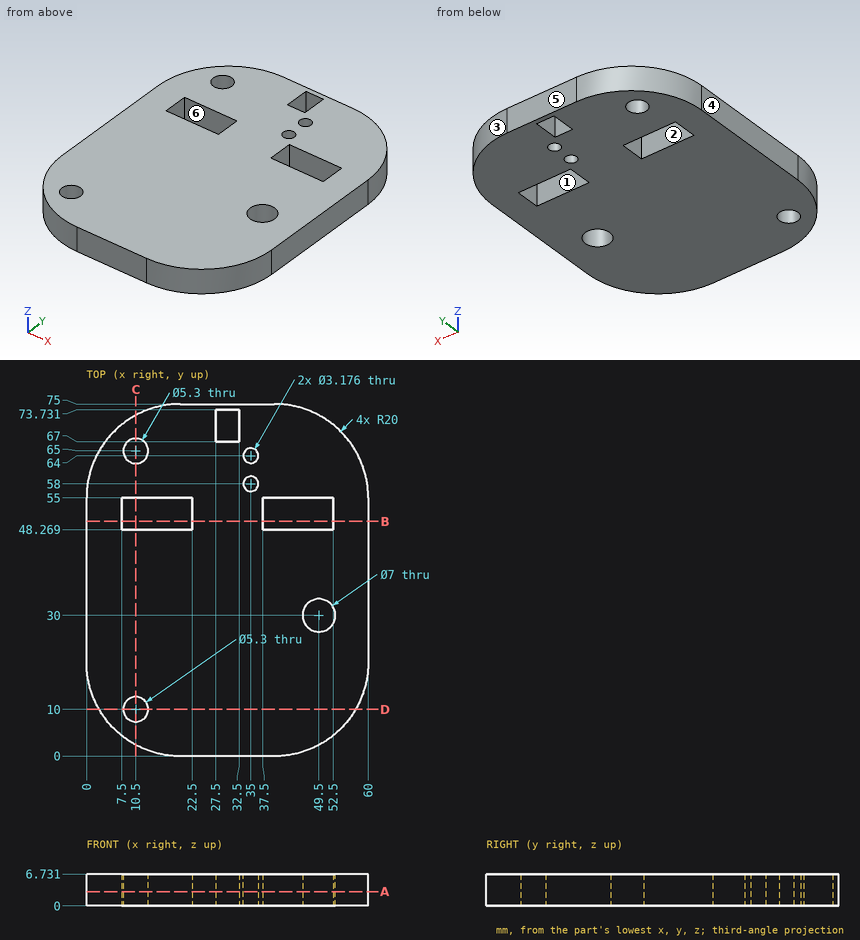
Answer from the drawing. Dimensions are ordinates in mm from the lowest x, y and z of the part. A direction names the side the tool comes from. Give positions to 0.01 mm unless a question says otherwise; leave off trailing zeros. Loops run counter-clockwise (first coordinate to the right, second up) from the corner with the lowest first, then second, coordinate; pieces in that order, holes last.
Item 1: For the marked faces 5 and 6, determine the directions among +Z, -Z, +X, -X, +Y, -Y from which every point of the face is accessible in a straight line to the end or side of a thin tool.
Item 2: The mould has two halves that part along Y. Classify the marked faces 1, 2, 3 and 4: released by +Y, released by -Y, zero draft, split by the parting line, or undercut.
Item 3: Each of these flat-tipped pins is pushed along its axis until it touches: pin 1 Ø2 at (x, z) = (44.5, 5) entering from +Y; pin 2 Ø2 at (x, z) = (45, 3.5) entering from +Y; pin 3 Ø2 at (x, z) = (13.5, 2.5) entering from +Y; pin 4 Ø3 at (x, y) = (10.5, 10) entering from +Z. Where does it stop, or does it pass through?
Item 4: The part is cut by section D-D (y = 10). Write down the section's boundary in (x, z), and give its area (3 significant figures).
Item 5: Find the intervals of material crossed by line 1 along Y through (x, z) = (35, 3.5); line 2 along X through (y, z) = (54, 1); line 3 along Y through (x, z) = (36, 4), in increasing order.
Item 6: The part is cut by section C-C (x = 10.5). Write down the section's boundary in (y, z), and give its area (3 significant figures).
Item 7: The part is cut by section B-B (y = 50). Write down the section's boundary in (x, z), and give its area (3 significant figures).
Item 8: The part is cut by section A-A (z = 3). Give the number of separate pieces and of enclosed holes in the cut face, and give its area (3 significant figures).
Taken from the geometry:
1. face 5: +Z, -Z, +X, -X, +Y
1. face 6: +Z, -Z
2. face 1: undercut
2. face 2: undercut
2. face 3: released by +Y
2. face 4: zero draft
3. pin 1: stops at y = 74.69
3. pin 2: stops at y = 74.6
3. pin 3: stops at y = 74.23
3. pin 4: passes through
4. outline: (2.68, 0) - (7.85, 0) - (7.85, 6.73) - (2.68, 6.73) - close; (13.15, 0) - (57.32, 0) - (57.32, 6.73) - (13.15, 6.73) - close
4. area: 332 mm2
5. line 1: y = 0 to 56.41, 59.59 to 62.41, 65.59 to 75
5. line 2: x = 0 to 7.5, 22.5 to 37.5, 52.5 to 60
5. line 3: y = 0 to 56.77, 59.23 to 62.77, 65.23 to 75
6. outline: (2.4, 0) - (7.35, 0) - (7.35, 6.73) - (2.4, 6.73) - close; (12.65, 0) - (48.27, 0) - (48.27, 6.73) - (12.65, 6.73) - close; (55, 0) - (62.35, 0) - (62.35, 6.73) - (55, 6.73) - close; (67.65, 0) - (72.6, 0) - (72.6, 6.73) - (67.65, 6.73) - close
6. area: 356 mm2
7. outline: (0, 0) - (7.5, 0) - (7.5, 6.73) - (0, 6.73) - close; (22.5, 0) - (37.5, 0) - (37.5, 6.73) - (22.5, 6.73) - close; (52.5, 0) - (60, 0) - (60, 6.73) - (52.5, 6.73) - close
7. area: 202 mm2
8. separate pieces: 1
8. enclosed holes: 8
8. area: 3,820 mm2
